Source: CAD feature listing. Evaluate the final solid. Frame: model axes, mm. A direction names the side the tool comes from. Round coordinates to 2 decimals unless told otherwise and drop trailing zeros. Order: outer loops, then holes, each group sorted by start corner. A loop starts at its lowest first (then second) coordinate and runs counter-clockwise, first axis right, second up. Notation, with made-up numbers: (25.25, -26) - (30.25, -26) arc R29 ccw to (30.25, 6) - close; hole circle Ø1 at (26, 59.25). An arc over 180 degrees is marked (long way). Return JSON: item names as keys, results as strings. Group by question number.
1) Ray query, line 1 (X direction, y = 6.7, z = 0); line 2 (Z direction, x = 0, y = 0.6). Return the intervals inside material, ascending. Write a range as from..to.
2) Section C-C, the plane z = 0. Return loops of the section in (x, y).
3) Contact query for a flat-ended pin moving along its axis: P1, Ø2.5, axis at x = 0.5, z = 1, coming from the +Y side. Output: stop coordinate, or through.
4) Section B-B, the plane y = 6.5. Return loops of the section in (x, z).
5) Access query for faces 4 (the cylindrical face through (-0.54, 7.01, 2.44)), 5 (the flat face through (3, 8, 0)), 6 (the cylindrical face through (-0.217, 0.493, -0.976)). Directions: +Z, -Z, +X, -X, +Y, -Y. A direction counts if a zero-diameter tool reaches every point of the face in a straight line with its end or side. Return the directions, or none.
6) Mould query, pull axis X, two halves, no side actions, for faces 1 (the flat face through (-6, 4, 0)), 2 (the flat face through (0, 6, 0)), 3 (the flat face through (0, 4, 6)). Classes: pulls with the +X half, pulls with the -X half, needs draft (parallel to the pull), parting line crosses it, or undercut.
7) Section A-A, the plane x = 0. Return loops of the section in (y, z).
8) Section D-D, the plane z = -1.5. Return loops of the section in (x, y), plus the area to 3 significant figures.
```python
from build123d import *

# Parameters (mm, degrees)
SKETCH1_W           = 12
SKETCH1_H           = 12
BOSS_EXTRUDE1_DEPTH = 8
SKETCH2_R           = 2.5
CUT_EXTRUDE1_DEPTH  = 2
SKETCH3_R           = 1
CUT_EXTRUDE2_DEPTH  = 2
FILLET1_R           = 1


with BuildPart() as part:
    # Sketch1 → Boss-Extrude1 (new body)
    with BuildSketch(Plane(origin=(0, 0, 0), x_dir=(1, 0, 0), z_dir=(0, 1, 0))):
        Rectangle(SKETCH1_W, SKETCH1_H)
    extrude(amount=BOSS_EXTRUDE1_DEPTH)

    # Sketch2 → Cut-Extrude1 (cut)
    with BuildSketch(Plane(origin=(0, 8, 0), x_dir=(1, 0, 0), z_dir=(0, 1, 0))):
        Circle(SKETCH2_R)
    extrude(amount=-CUT_EXTRUDE1_DEPTH, mode=Mode.SUBTRACT)

    # Sketch3 → Cut-Extrude2 (cut)
    with BuildSketch(Plane.XZ):
        Circle(SKETCH3_R)
    extrude(amount=-CUT_EXTRUDE2_DEPTH, mode=Mode.SUBTRACT)

    # Fillet1
    fillet1_edges = [part.edges().sort_by_distance(p)[0] for p in [
        (-1, 2, 0),
    ]]
    fillet(fillet1_edges, radius=FILLET1_R)


solid = part.part
```
Geometry check:
{
 "1": {"line 1": "-6..-2.5, 2.5..6", "line 2": "-6..-1, 1..6"},
 "2": {"outline": "(-6, 0) - (-1, 0) - (-1, 1) arc R1 cw to (1, 1) - (1, 0) - (6, 0) - (6, 8) - (2.5, 8) - (2.5, 6) - (-2.5, 6) - (-2.5, 8) - (-6, 8) - close"},
 "3": {"P1": "y = 6"},
 "4": {"outline": "(-6, -6) - (6, -6) - (6, 6) - (-6, 6) - close; hole circle Ø5 at (0, 0)"},
 "5": {"face 4": "+Y", "face 5": "+Z, -Z, +X, -X, +Y", "face 6": "-Y"},
 "6": {"face 1": "pulls with the -X half", "face 2": "undercut", "face 3": "needs draft"},
 "7": {"outline": "(0, -6) - (8, -6) - (8, -2.5) - (6, -2.5) - (6, 2.5) - (8, 2.5) - (8, 6) - (0, 6) - (0, 1) - (1, 1) arc R1 cw to (1, -1) - (0, -1) - close"},
 "8": {"outline": "(-6, 0) - (6, 0) - (6, 8) - (2, 8) - (2, 6) - (-2, 6) - (-2, 8) - (-6, 8) - close", "area": "88.0 mm2"}
}
